The figure shows three views and two pictorial views of one solid part (mm, origin at its lowest corner). Answer the questions. Give positions to 0.01 mm unless a question says otherwise; leave off trailing zeros. Loops run counter-clockwise (first coordinate to the right, second up) from the corner with the lowest first, then second, coordinate; pieces in that order, holes last. Notation, with made-up numbers: (43, 60.5) -> (66, 60.5) arc R6 ccw to (66, 65.5) -> close; hole circle Ø8 at (-7.75, 48.25). An arc over 180 degrees is marked (long way). Answer as CSV lines item,"result". Start each with the question number.
1. Find the intervals of material crossed by line 1 along Y through (x, z) = (37.5, 6.25); line 2 along X through (y, z) = (48, 4.5); line 3 along Y through (x, z) = (7.5, 4.5), in increasing order.
2. Flat-ended cylindrical pins translate along their axes: pin 1 Ø1.5 at (y, z) = (28.5, 3) entering from -X; pin 2 Ø2 at (y, z) = (11, 7) entering from +X; pin 3 Ø1.5 at (x, z) = (54.5, 7) entering from +Y. Find the tip coordinate at first contact, or state that the pin passes through.
3. Find section C-C, the plane x = 37.5. Give the vertices of the cut face in (y, z).
4. Determine the mould class of the marked faces 1, 2 and 3 for opening direction X: +X half, -X half, draft (parallel to the pull), parting line (faces both ways), or undercut.
5. Find section D-D, the plane z = 1.75. Give the vertices of the cut face in (x, y), and give its area (3 significant figures).
6. Find section A-A, the plane x = 7.5. Give the vertices of the cut face in (y, z).
7. Find section B-B, the plane y = 37.5. Give the vertices of the cut face in (x, z), and give its area (3 significant figures).
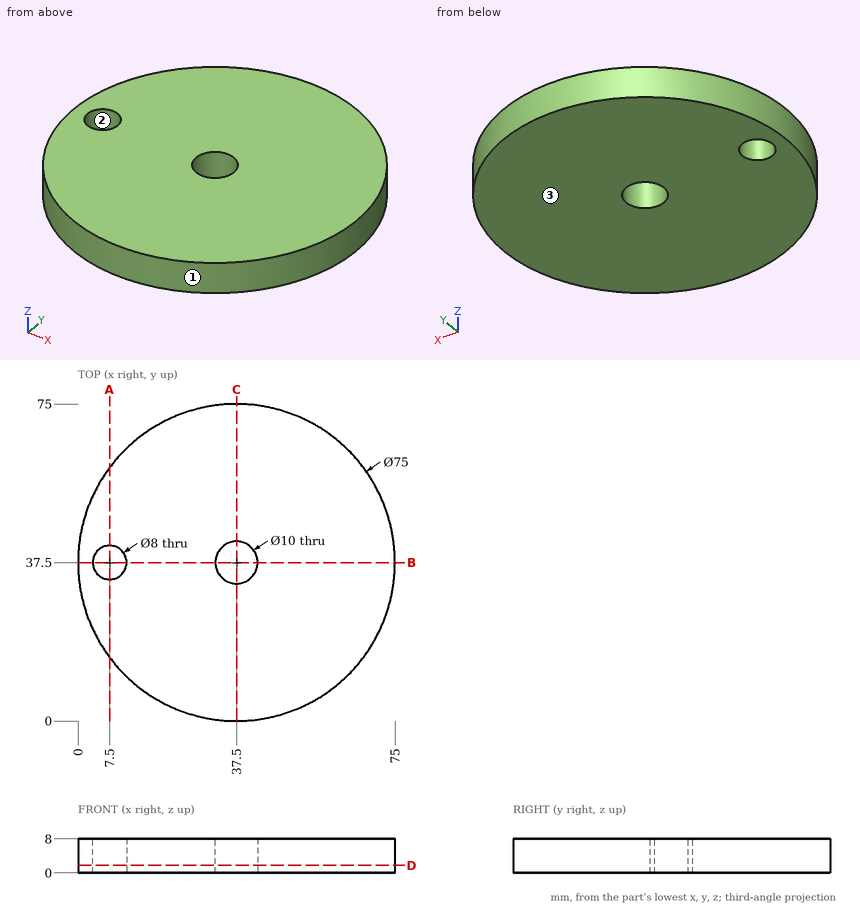
Resolved:
1,line 1,"y = 0 to 32.5, 42.5 to 75"
1,line 2,"x = 1.5 to 73.5"
1,line 3,"y = 15 to 33.5, 41.5 to 60"
2,pin 1,"stops at x = 0.92"
2,pin 2,"stops at x = 65"
2,pin 3,"stops at y = 71.3"
3,outline,"(0, 0) -> (32.5, 0) -> (32.5, 8) -> (0, 8) -> close; (42.5, 0) -> (75, 0) -> (75, 8) -> (42.5, 8) -> close"
4,face 1,"parting line"
4,face 2,"undercut"
4,face 3,"draft"
5,outline,"circle Ø75 at (37.5, 37.5); hole circle Ø8 at (7.5, 37.5); hole circle Ø10 at (37.5, 37.5)"
5,area,"4,290 mm^2"
6,outline,"(15, 0) -> (33.5, 0) -> (33.5, 8) -> (15, 8) -> close; (41.5, 0) -> (60, 0) -> (60, 8) -> (41.5, 8) -> close"
7,outline,"(0, 0) -> (3.5, 0) -> (3.5, 8) -> (0, 8) -> close; (11.5, 0) -> (32.5, 0) -> (32.5, 8) -> (11.5, 8) -> close; (42.5, 0) -> (75, 0) -> (75, 8) -> (42.5, 8) -> close"
7,area,"456 mm^2"
